Autodesk Fusion 360 part; units mm, degrees
sketch "Sketch1" plane through (0, 0, 0) normal (0, 1, 0) x (1, 0, 0)
  line L0 (0, 20) -> (20, 20)
  line L1 (20, 0) -> (0, 0)
  line L2 (0, 20) -> (0, 0)
  line L3 (10, 11.15) -> (10, 8.65)
  line L4 (20, 20) -> (20, 18)
  line L5 (20, 18) -> (10, 11.15)
  line L6 (10, 8.65) -> (20, 2)
  line L7 (20, 2) -> (20, 0)
  dimension "d3" = 20
  dimension "d4" = 20
  dimension "d5" = 10
  dimension "d7" = 2
  dimension "d9" = 2.5
  dimension "d18" = 8.85
revolve "Revolve1" add sketch "Sketch1" angle 360 about axis through (0, 0, 1.75) along (0, 0, 1)
hole "Hole1" at (-0.0164, -0.0454, 0) direction (0, 0, -1) diameter 8 depth 15 tip angle 180
sketch "Sketch2" plane through (0, 0, 0) normal (0, 0, 1) x (1, 0, 0)
sketch "Sketch3" plane through (0, 0, -15) normal (0, 0, 1) x (1, 0, 0)
  circle A0 centre (-0.0164, -0.0454) radius 4
  circle A1 centre (-0.0164, -0.0454) radius 1.5
  dimension "d15" = 3
extrude "Extrude1" cut sketch "Sketch3" against normal blind 17 contours A1
sketch "Sketch4" plane through (0, 0, -20) normal (0, 0, -1) x (-1, 0, 0)
  circle A0 centre (0, 0) radius 20
  circle A1 centre (0, 0) radius 3.5
  circle A2 centre (0.0164, -0.0454) radius 1.5
  dimension "d19" = 7
extrude "Extrude2" cut sketch "Sketch4" against normal blind 3 contours A1 | A2
sketch "Sketch5" plane through (0, 0, 0) normal (0, 1, 0) x (1, 0, 0)
  line L0 (-1.7235, 9.4108) -> (1.7051, 9.4108)
  line L1 (1.7051, 9.4108) -> (1.7051, 10.3321)
  line L2 (1.7051, 10.3321) -> (-1.7235, 10.3321)
  line L3 (-1.7235, 10.3321) -> (-1.7235, 9.4108)
extrude "Extrude3" cut sketch "Sketch5" along normal blind 30 and the other way blind 15
Source: CAD feature listing. Evaluate the final solid. Frame: model axes, mm. A direction names the side the tool comes from. Give positions to 0.01 mm unless a question says otherwise; leave off trailing zeros. Write each loop counter-clockwise with the first axis right and the second up, starting at its lowest first coordinate (ties: lowest second). Pieces come first, ordered by that corner, then holes. Notation, with made-up numbers: M -24.5,79.5 L 34.5,79.5 A19 cw 34.5,99.5 Z; hole C 12,13.5 d11. An arc over 180 degrees is marked long. Return JSON: item names as keys, results as strings. Group by question number.
1) Set-up query: faces 1 (the face through (0, 7, -9.411)), 2 (the face through (-3.233, -1.341, -18.521)), 3 (the face through (-0.19, 3.95, -7.6)), 4 (the face through (-2.17, -9.76, -9.88)), 5 (the face through (-4.336, -19.524, -18.986)). Return all of +Z, -Z, +X, -X, +Y, -Y with unobstructed straight access to the full face (end or side cutting, diameter ignored); none if empty.
2) Pull-direction query (Y, two-part tool) for faces 6 (the face through (0, -2, -15)), 7 (the face through (10.135, 3.192, -8.234)), 8 (the face through (0, -7, -9.411)), 9 (the face through (-1, -2, -17)); classes: pulls with the +Y half, pulls with the -Y half, needs draft (parallel to the pull), parting line crosses it, or undercut.
3) Cut plane A-A, the plane z = -13.25. Output: boundary loops of the cut face in (x, y), plus the area to 3 significant figures.
4) Material intervals for line 1 along Y through (x, z) = (0, -16); line 2 along Z through (x, y) = (-12, -13.5); line 3 along Z through (x, y) = (-8, -8.5), sorted ascending. Write a range as [from, to].
5) Pin query (flat end, axial travel): P1, Ø2.5, axis at x = -1.5, y = -1, coming from the +Z side; P2, Ø2, axis at x = -1, z = -7, coming from the -Y side; P3, Ø8, axis at y = -3.5, z = -12.5, coming from the -X side. Return the tip coordinate at first contact, or that it passes through.
Recorded:
{
 "1": {"face 1": "+Y, -Y", "face 2": "-Z", "face 3": "+Z", "face 4": "none", "face 5": "+Z, -Z"},
 "2": {"face 6": "undercut", "face 7": "parting line crosses it", "face 8": "needs draft", "face 9": "undercut"},
 "3": {"outline": "C 0,0 d26.13; hole C -0.02,-0.05 d8", "area": "486 mm²"},
 "4": {"line 1": "y = [-17.08, -1.55], [1.45, 17.08]", "line 2": "z = [-20, -16.67], [-3.29, 0]", "line 3": "z = [-20, -12.3], [-7.54, 0]"},
 "5": {"P1": "stops at z = -15", "P2": "stops at y = -13.95", "P3": "stops at x = -17.51"}
}
